from build123d import *

# Parameters (mm, degrees)
ESQUISSE1_W        = 5
ESQUISSE1_H        = 25
BOSS_EXTRU_1_DEPTH = 83.80285333
CONG_1_R           = 4
D_GAGEMENT_M31_D   = 3.4


with BuildPart() as part:
    # Esquisse1 → Boss.-Extru.1 (new body)
    with BuildSketch(Plane.XY):
        with Locations((2.5, 0)):
            Rectangle(ESQUISSE1_W, ESQUISSE1_H)
    extrude(amount=BOSS_EXTRU_1_DEPTH)

    # Congé1
    cong_1_edges = [part.edges().sort_by_distance(p)[0] for p in [
        (2.5, -12.5, 83.80285333),
        (2.5, 12.5, 83.80285333),
        (2.5, -12.5, 0),
        (2.5, 12.5, 0),
    ]]
    fillet(cong_1_edges, radius=CONG_1_R)

    # Dégagement M31 (through all)
    with Locations(Plane(origin=(5, 0, 0), x_dir=(0, 0, -1), z_dir=(1, 0, 0))):
        with Locations((-4.5, -8), (-4.5, 8), (-20.5, 8), (-63.30285333, 8), (-79.30285333, 8), (-79.30285333, -8), (-63.30285333, -8), (-20.5, -8)):
            Hole(D_GAGEMENT_M31_D / 2)


solid = part.part
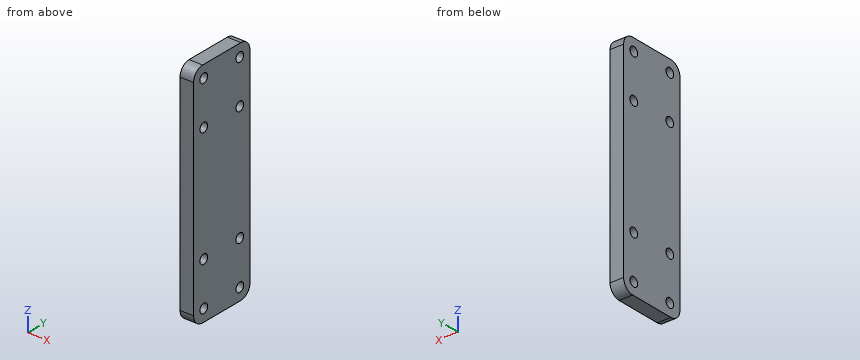
CAD build for the part. Positions are in the model's coordinates, mm. Give positions to 0.01 mm unless a question says otherwise; leave off trailing zeros. Loops run counter-clockwise (first coordinate to the right, second up) from the corner with the lowest first, then second, coordinate; pieces in that order, holes last. Notation, with made-up numbers: M 52,77 L 80,77 A8 ccw 80,92 Z; hole C 43.25,-34.5 d4. An arc over 180 degrees is marked long. Answer in a Markdown table with one row per item. Add a question column.
Item 1: Probe probe 1 along Y at (x, z) = (2, 4.5); probe 2 along Z at (x, y) = (0.8, -8.5); probe 3 along Z at (x, y) = (2.55, 9.25). List the from-to ranges inside material, lowest first.
Item 2: Band-saw the part on A-A on x = 1.35. Give the number of separate pieces and of enclosed holes in the cut face, then the cut area to 3 significant figures.
Item 3: Band-saw the part on B-B on z = 20.5. Give the cut face in (x, y).
Reply:
| question | item | result |
|---|---|---|
| 1 | probe 1 | y = -12.5 to -9.7, -6.3 to 6.3, 9.7 to 12.5 |
| 1 | probe 2 | z = 0 to 2.88, 6.12 to 18.88, 22.12 to 61.68, 64.93 to 77.68, 80.93 to 83.8 |
| 1 | probe 3 | z = 0.07 to 3.35, 5.65 to 19.35, 21.65 to 62.15, 64.46 to 78.15, 80.46 to 83.73 |
| 2 | separate pieces | 1 |
| 2 | enclosed holes | 8 |
| 2 | area | 2,010 mm^2 |
| 3 | outline | M 0,-12.5 L 5,-12.5 L 5,-9.7 L 0,-9.7 Z; M 0,-6.3 L 5,-6.3 L 5,6.3 L 0,6.3 Z; M 0,9.7 L 5,9.7 L 5,12.5 L 0,12.5 Z |
